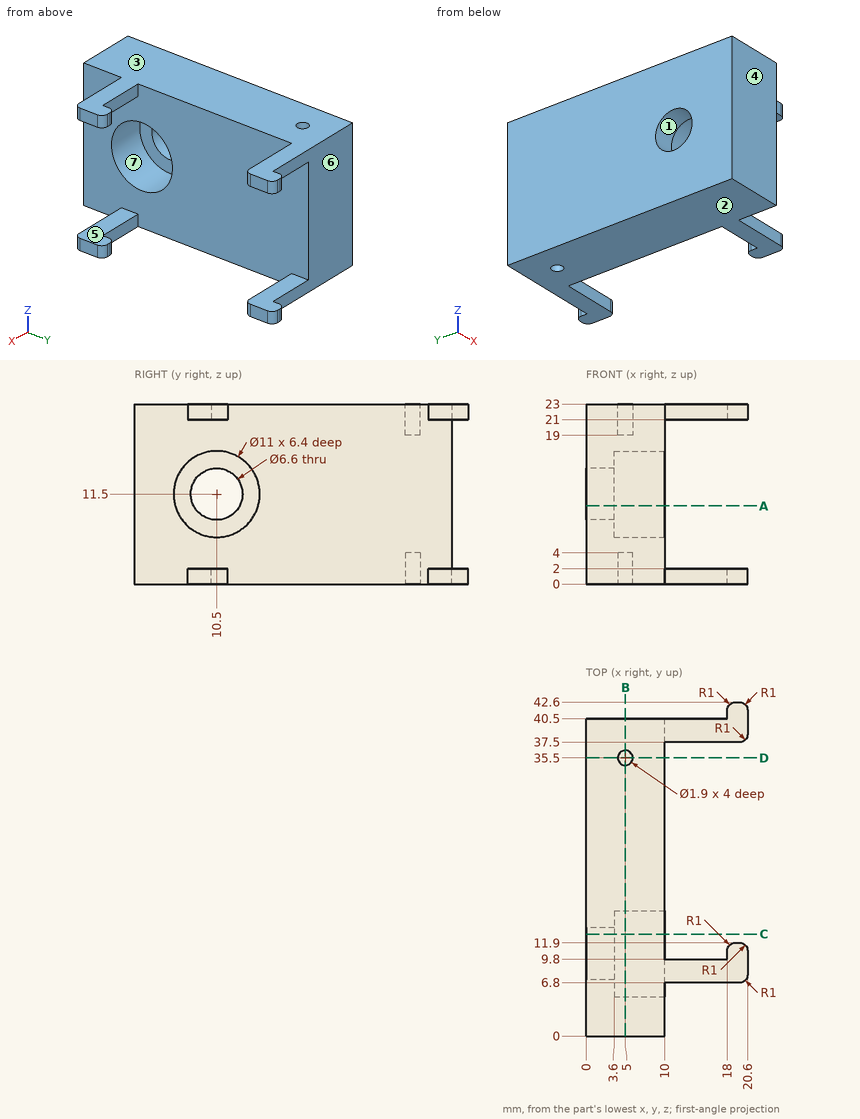
Here's the drawing with two shaded views (mm, measured from the low corner). I have some questions. A direction names the side the tool comes from. Coordinates: 2 decimals unless noted, no trailing zeros. Order: outer loops, then holes, each group sorted by start corner. A loop starts at its lowest first (then second) coordinate and runs counter-clockwise, first axis right, second up. Notation, with made-up numbers: (-3, 71.25) -> (24, 71.25) arc R14 cw to (24, 75.25) -> close; hole circle Ø10 at (-16.75, 83.25). An arc over 180 degrees is marked (long way). One line per question, with ' | ' between items.
Q1. Imagine slicing it at A-A on z = 10. Please give me the cut outline in (x, y).
Return value:
outline: (0, 0) -> (10, 0) -> (10, 5.21) -> (3.6, 5.21) -> (3.6, 7.56) -> (0, 7.56) -> close; (0, 13.44) -> (3.6, 13.44) -> (3.6, 15.79) -> (10, 15.79) -> (10, 40.5) -> (0, 40.5) -> close
Q2. Thinking about a two-plate mould opening in Z: for the marked faces 1, 2, 3 and 4, which applies, pulls with the +Z half, pulls with the -Z half, needs draft (parallel to the pull), parting line crosses it, or undercut?
Return value:
face 1: undercut | face 2: pulls with the -Z half | face 3: pulls with the +Z half | face 4: needs draft
Q3. Imagine slicing it at D-D on y = 35.5. Please give me the cut outline in (x, z).
Return value:
outline: (0, 0) -> (4.05, 0) -> (4.05, 4) -> (5.95, 4) -> (5.95, 0) -> (10, 0) -> (10, 23) -> (5.95, 23) -> (5.95, 19) -> (4.05, 19) -> (4.05, 23) -> (0, 23) -> close
Q4. Imagine slicing it at C-C on y = 13. Please give me the cut outline in (x, z).
Return value:
outline: (0, 0) -> (10, 0) -> (10, 6.6) -> (3.6, 6.6) -> (3.6, 9.35) -> (0, 9.35) -> close; (0, 13.65) -> (3.6, 13.65) -> (3.6, 16.4) -> (10, 16.4) -> (10, 23) -> (0, 23) -> close
Q5. I'm going to push flat-ended pins straight in: P1, Ø4, axis at x = 15.5, y = 41.5, coming from the -Z side; P2, Ø1, axis at x = 14, z = 1, coming from the -Y side; P3, Ø1.6, axis at x = 13, z = 1, coming from the +Y side; P4, Ø1, axis at y = 32, z = 17, coming from the +X side. Where does each tip first touch, or does it pass through?
Return value:
P1: z = 0 | P2: y = 6.8 | P3: y = 40.5 | P4: x = 10
Q6. If I drill on L1, parallel to Y at x = 5, z = 21.05; L2, parallel to Z at x = 17, y = 8; L3, parallel to X at y = 35.5, z = 21.8, over which ranges is the centre line in solid material (lowest first)?
Return value:
L1: 0 to 34.55, 36.45 to 40.5 | L2: 0 to 2, 21 to 23 | L3: 0 to 4.05, 5.95 to 10
Q7. On a 3-axis mill with a long thin cutter (end or side, diameter ignored), from which of +Z, -Z, +X, -X, +Y, -Y can I reach the whole of each face in a straight line? I mean the marked faces 5, 6 and 7. Say none if no direction works.
Return value:
face 5: +X, +Y, -Y | face 6: +Z, -Z, -X, +Y | face 7: +X
Q8. Imagine slicing it at B-B on x = 5. Please give me the cut outline in (y, z), and give its area (3 significant figures).
Return value:
outline: (0, 0) -> (34.55, 0) -> (34.55, 4) -> (36.45, 4) -> (36.45, 0) -> (40.5, 0) -> (40.5, 23) -> (36.45, 23) -> (36.45, 19) -> (34.55, 19) -> (34.55, 23) -> (0, 23) -> close; hole circle Ø11 at (10.5, 11.5) | area: 821 mm²
